```python
from build123d import *

# Parameters (mm, degrees)
SKETCH_1_R          = 2.55
EXTRUDE_1_DEPTH     = 10
SKETCH_2_W          = 40
SKETCH_2_H          = 20
EXTRUDE_2_DEPTH     = 3
EXTRUDE_3_DEPTH     = 3
CUT_EXTRUDE_1_DEPTH = 10
SKETCH_5_R          = 3
CUT_EXTRUDE_2_DEPTH = 10
SKETCH_6_R          = 3
SKETCH_6_R_2        = 4.25
EXTRUDE_4_DEPTH     = 3
FILLET_1_R          = 1.5
SKETCH_7_R          = 6
SKETCH_7_R_2        = 3
EXTRUDE_5_DEPTH     = 5
SKETCH_8_R          = 8.25
EXTRUDE_6_DEPTH     = 5
FILLET_3_R          = 1.5


with BuildPart() as part:
    # 草图1 → 凸台-拉伸1 (new body)
    with BuildSketch(Plane.XY):
        Polygon((-20, 0), (-20, -6.9), (-18.2, -6.9), (-18.2, -4.5), (-16.560660172, -4.5), (-13.9, -7.160660172), (-13.9, -12.839339828), (-16.560660172, -15.5), (-18.2, -15.5), (-18.2, -13.1), (-20, -13.1), (-20, -20), (-13.1, -20), (-13.1, -18.2), (-15.5, -18.2), (-15.5, -16.560660172), (-12.839339828, -13.9), (-7.160660172, -13.9), (-4.5, -16.560660172), (-4.5, -18.2), (-6.9, -18.2), (-6.9, -20), (0, -20), (6.9, -20), (6.9, -18.2), (4.5, -18.2), (4.5, -16.560660172), (7.160660172, -13.9), (12.839339828, -13.9), (15.5, -16.560660172), (15.5, -18.2), (13.1, -18.2), (13.1, -20), (20, -20), (20, -13.1), (18.2, -13.1), (18.2, -15.5), (16.560660172, -15.5), (13.9, -12.839339828), (13.9, -7.160660172), (16.560660172, -4.5), (18.2, -4.5), (18.2, -6.9), (20, -6.9), (20, 0), (13.1, 0), (13.1, -1.8), (15.5, -1.8), (15.5, -3.439339828), (12.839339828, -6.1), (7.160660172, -6.1), (4.5, -3.439339828), (4.5, -1.8), (6.9, -1.8), (6.9, 0), (0, 0), (-6.9, 0), (-6.9, -1.8), (-4.5, -1.8), (-4.5, -3.439339828), (-7.160660172, -6.1), (-12.839339828, -6.1), (-15.5, -3.439339828), (-15.5, -1.8), (-13.1, -1.8), (-13.1, 0), align=None)
        with Locations((-10, -10)):
            Circle(SKETCH_1_R, mode=Mode.SUBTRACT)
        with Locations((10, -10)):
            Circle(SKETCH_1_R, mode=Mode.SUBTRACT)
        Polygon((-3.439339828, -4.5), (-6.1, -7.160660172), (-6.1, -12.839339828), (-3.439339828, -15.5), (-3.439339828, -18.2), (3.439339828, -18.2), (3.439339828, -15.5), (6.1, -12.839339828), (6.1, -7.160660172), (3.439339828, -4.5), (3.439339828, -1.8), (-3.439339828, -1.8), align=None, mode=Mode.SUBTRACT)
    extrude(amount=EXTRUDE_1_DEPTH)

    # 草图2 → 凸台-拉伸2 (add)
    with BuildSketch(Plane.XY.offset(10)):
        with Locations((0, -10)):
            Rectangle(SKETCH_2_W, SKETCH_2_H)
    extrude(amount=EXTRUDE_2_DEPTH)

    # 草图3 → 凸台-拉伸3 (add)
    with BuildSketch(Plane(origin=(0, 0, 10), x_dir=(-1, 0, 0), z_dir=(0, 0, -1))):
        Polygon((-13.1, -20), (-6.9, -20), (-6.9, -18.2), (-4.5, -18.2), (-4.5, -16.560660172), (-7.160660172, -13.9), (-12.839339828, -13.9), (-15.5, -16.560660172), (-15.5, -18.2), (-13.1, -18.2), align=None)
        Polygon((-20, -6.9), (-20, -13.1), (-18.2, -13.1), (-18.2, -15.5), (-16.560660172, -15.5), (-13.9, -12.839339828), (-13.9, -7.160660172), (-16.560660172, -4.5), (-18.2, -4.5), (-18.2, -6.9), align=None)
        Polygon((-6.9, 0), (-13.1, 0), (-13.1, -1.8), (-15.5, -1.8), (-15.5, -3.439339828), (-12.839339828, -6.1), (-7.160660172, -6.1), (-4.5, -3.439339828), (-4.5, -1.8), (-6.9, -1.8), align=None)
        Polygon((6.9, -20), (13.1, -20), (13.1, -18.2), (15.5, -18.2), (15.5, -16.560660172), (12.839339828, -13.9), (7.160660172, -13.9), (4.5, -16.560660172), (4.5, -18.2), (6.9, -18.2), align=None)
        Polygon((20, -13.1), (20, -6.9), (18.2, -6.9), (18.2, -4.5), (16.560660172, -4.5), (13.9, -7.160660172), (13.9, -12.839339828), (16.560660172, -15.5), (18.2, -15.5), (18.2, -13.1), align=None)
        Polygon((13.1, 0), (6.9, 0), (6.9, -1.8), (4.5, -1.8), (4.5, -3.439339828), (7.160660172, -6.1), (12.839339828, -6.1), (15.5, -3.439339828), (15.5, -1.8), (13.1, -1.8), align=None)
    extrude(amount=EXTRUDE_3_DEPTH)

    # 草图4 → 切除-拉伸1 (cut)
    with BuildSketch(Plane(origin=(0, 0, 0), x_dir=(-1, 0, 0), z_dir=(0, 0, -1))):
        Polygon((6.9, 0), (-6.9, 0), (-6.9, -1.8), (-4.5, -1.8), (-4.5, -3.439339828), (-7.160660172, -6.1), (-12.839339828, -6.1), (-15.5, -3.439339828), (-15.5, -1.8), (-13.1, -1.8), (-13.1, 0), (-20, 0), (-20, -6.9), (-18.2, -6.9), (-18.2, -4.5), (-16.560660172, -4.5), (-13.9, -7.160660172), (-13.9, -12.839339828), (-16.560660172, -15.5), (-18.2, -15.5), (-18.2, -13.1), (-20, -13.1), (-20, -20), (-13.1, -20), (-13.1, -18.2), (-15.5, -18.2), (-15.5, -16.560660172), (-12.839339828, -13.9), (-7.160660172, -13.9), (-4.5, -16.560660172), (-4.5, -18.2), (-6.9, -18.2), (-6.9, -20), (6.9, -20), (6.9, -18.2), (4.5, -18.2), (4.5, -16.560660172), (7.160660172, -13.9), (12.839339828, -13.9), (15.5, -16.560660172), (15.5, -18.2), (13.1, -18.2), (13.1, -20), (20, -20), (20, -13.1), (18.2, -13.1), (18.2, -15.5), (16.560660172, -15.5), (13.9, -12.839339828), (13.9, -7.160660172), (16.560660172, -4.5), (18.2, -4.5), (18.2, -6.9), (20, -6.9), (20, 0), (13.1, 0), (13.1, -1.8), (15.5, -1.8), (15.5, -3.439339828), (12.839339828, -6.1), (7.160660172, -6.1), (4.5, -3.439339828), (4.5, -1.8), (6.9, -1.8), align=None)
    extrude(amount=-CUT_EXTRUDE_1_DEPTH, mode=Mode.SUBTRACT)

    # 草图5 → 切除-拉伸2 (cut)
    with BuildSketch(Plane(origin=(0, 0, 10), x_dir=(-1, 0, 0), z_dir=(0, 0, -1))):
        with Locations((-10, -10)):
            Circle(SKETCH_5_R)
        with Locations((10, -10)):
            Circle(SKETCH_5_R)
    extrude(amount=-CUT_EXTRUDE_2_DEPTH, mode=Mode.SUBTRACT)

    # 草图6 → 凸台-拉伸4 (add)
    with BuildSketch(Plane.XY.offset(13)):
        Polygon((-20, 0), (20, 0), (20, 35), (0, 35), (-20, 35), align=None)
        with Locations((-10, 10.36)):
            Circle(SKETCH_6_R, mode=Mode.SUBTRACT)
        with Locations((10, 10.36)):
            Circle(SKETCH_6_R, mode=Mode.SUBTRACT)
        with Locations((0, 25)):
            Circle(SKETCH_6_R_2, mode=Mode.SUBTRACT)
    extrude(amount=-EXTRUDE_4_DEPTH)

    # 圆角1
    fillet_1_edges = [part.edges().sort_by_distance(p)[0] for p in [
        (20, -20, 11.5),
        (-20, -20, 11.5),
        (-20, 35, 11.5),
        (20, 35, 11.5),
    ]]
    fillet(fillet_1_edges, radius=FILLET_1_R)

    # 草图7 → 凸台-拉伸5 (add)
    # profile 1 of 2: a face of its own
    with BuildSketch(Plane(origin=(0, 0, 10), x_dir=(-1, 0, 0), z_dir=(0, 0, -1))):
        with Locations(Location((-10, 10.36, 0), (0, 0, 180))):
            Circle(SKETCH_7_R)
        with Locations(Location((-10, 10.36, 0), (0, 0, 180))):
            Circle(SKETCH_7_R_2, mode=Mode.SUBTRACT)
    # profile 2 of 2: a face of its own
    with BuildSketch(Plane(origin=(0, 0, 10), x_dir=(-1, 0, 0), z_dir=(0, 0, -1))):
        with Locations(Location((10, 10.36, 0), (0, 0, 180))):
            Circle(SKETCH_7_R)
        with Locations(Location((10, 10.36, 0), (0, 0, 180))):
            Circle(SKETCH_7_R_2, mode=Mode.SUBTRACT)
    extrude(amount=EXTRUDE_5_DEPTH)

    # 草图8 → 凸台-拉伸6 (add)
    with BuildSketch(Plane(origin=(0, 0, 10), x_dir=(-1, 0, 0), z_dir=(0, 0, -1))):
        with BuildLine():
            Line((-4.582575695, 35), (4.582575695, 35))
            ThreePointArc((4.582575695, 35), (0, 14), (-4.582575695, 35))
        make_face()
        with Locations((0, 25)):
            Circle(SKETCH_8_R, mode=Mode.SUBTRACT)
    extrude(amount=EXTRUDE_6_DEPTH)

    # 圆角3
    # the kernel refuses this fillet: 1.5 mm, written as the material it adds along each edge
    with BuildSketch(Plane(origin=(10, 10.36, 10), x_dir=(1, 0, 0), z_dir=(0, 1, 0))) as fillet_3_piece_1:
        with BuildLine():
            CenterArc((6 + FILLET_3_R, FILLET_3_R), FILLET_3_R, 180, 90)
            Line((6, FILLET_3_R), (6 - FILLET_3_R * 0.02, FILLET_3_R))
            Line((6 - FILLET_3_R * 0.02, FILLET_3_R), (6 - FILLET_3_R * 0.02, -FILLET_3_R * 0.02))
            Line((6 - FILLET_3_R * 0.02, -FILLET_3_R * 0.02), (6 + FILLET_3_R, -FILLET_3_R * 0.02))
            Line((6 + FILLET_3_R, -FILLET_3_R * 0.02), (6 + FILLET_3_R, 0))
        make_face()
    revolve(axis=Axis((10, 10.36, 10), (0, 0, -1)))
    with BuildSketch(Plane(origin=(-10, 10.36, 10), x_dir=(1, 0, 0), z_dir=(0, 1, 0))) as fillet_3_piece_2:
        with BuildLine():
            CenterArc((6 + FILLET_3_R, FILLET_3_R), FILLET_3_R, 180, 90)
            Line((6, FILLET_3_R), (6 - FILLET_3_R * 0.02, FILLET_3_R))
            Line((6 - FILLET_3_R * 0.02, FILLET_3_R), (6 - FILLET_3_R * 0.02, -FILLET_3_R * 0.02))
            Line((6 - FILLET_3_R * 0.02, -FILLET_3_R * 0.02), (6 + FILLET_3_R, -FILLET_3_R * 0.02))
            Line((6 + FILLET_3_R, -FILLET_3_R * 0.02), (6 + FILLET_3_R, 0))
        make_face()
    revolve(axis=Axis((-10, 10.36, 10), (0, 0, -1)))
    with BuildSketch(Plane(origin=(0, 25, 10), x_dir=(-0.08704252820230896, 0.9962045965985854, 0), z_dir=(0.9962045965985854, 0.08704252820230896, 0))) as fillet_3_piece_3_section:
        with BuildLine():
            CenterArc((11 + FILLET_3_R, -FILLET_3_R), FILLET_3_R, 90, 90)
            Line((11, -FILLET_3_R), (11 - FILLET_3_R * 0.02, -FILLET_3_R))
            Line((11 - FILLET_3_R * 0.02, -FILLET_3_R), (11 - FILLET_3_R * 0.02, FILLET_3_R * 0.02))
            Line((11 - FILLET_3_R * 0.02, FILLET_3_R * 0.02), (11 + FILLET_3_R, FILLET_3_R * 0.02))
            Line((11 + FILLET_3_R, FILLET_3_R * 0.02), (11 + FILLET_3_R, 0))
        make_face()
    fillet_3_piece_3 = revolve(axis=Axis((0, 25, 10), (0, 0, 1)), revolution_arc=350.013022923, mode=Mode.PRIVATE)
    fillet_3_piece_3 = split(fillet_3_piece_3, bisect_by=Plane(origin=(0, 35, 9.583684296), z_dir=(0, -1, 0)), keep=Keep.TOP, mode=Mode.PRIVATE)
    add(fillet_3_piece_3)


solid = part.part
```
Input: part model. Units: mm. Frame: model coordinates. A direction names the side the tool comes from. Coordinates: 2 decimals unless noted, no trailing zeros. Loops run counter-clockwise (first coordinate to the right, second up) from the corner with the lowest first, then second, coordinate; pieces in that order, holes last. Notation, with made-up numbers: M 43,4.5 L 90,4.5 A15 cw 90,8.5 Z; hole C -39.75,57.5 d8. An arc over 180 degrees is marked long. One line per item, written item: value.
(1) Reachability of faces 1 (the flat face through (18.2, -6, 8)), 2 (the flat face through (-6.9, -1, 8)), 3 (the flat face through (10, -3, 7)) from +Z, -Z, +X, -X, +Y, -Y: full face, straight path, thin tool, end or side. Return the list, or none.
Filled in:
face 1: -Z, +X, +Y
face 2: -Z
face 3: -Z, +X, -X, -Y
(2) Section A-A (y = -10). Output: boundary loops of the cut face in (x, z).
Filled in:
outline: M -20,7 L -13.9,7 L -13.9,10 L -13,10 L -13,13 L -20,13 Z; M -7,10 L 7,10 L 7,13 L -7,13 Z; M 13,10 L 13.9,10 L 13.9,7 L 20,7 L 20,13 L 13,13 Z
(3) Section D-D (z = 12). Output: boundary loops of the cut face in (x, y), and give its area (3 significant figures).
Filled in:
outline: M -20,-18.5 A1.5 ccw -18.5,-20 L 18.5,-20 A1.5 ccw 20,-18.5 L 20,33.5 A1.5 ccw 18.5,35 L -18.5,35 A1.5 ccw -20,33.5 Z; hole C -10,-10 d6; hole C -10,10.36 d6; hole C 0,25 d8.5; hole C 10,-10 d6; hole C 10,10.36 d6
area: 2,030 mm^2
(4) Pin query (flat end, axial travel): pin 1 (12 mm diameter, centred on x = 0.5, y = 24.5, fed in from -Z); pin 2 (6.5 mm diameter, centred on x = 17, y = -12.5, fed in from -Z); pin 3 (1.3 mm diameter, centred on x = 17.5, z = 9, fed in from -Y). Return the tip coordinate at first contact, or that it passes through.
Filled in:
pin 1: z = 10
pin 2: z = 7
pin 3: y = -15.5
(5) Section C-C (y = 25). Output: boundary loops of the cut face in (x, z).
Filled in:
outline: M -20,10 L -12.5,10 A1.5 cw -11,8.5 L -11,5 L -8.25,5 L -8.25,10 L -4.25,10 L -4.25,13 L -20,13 Z; M 4.25,10 L 8.25,10 L 8.25,5 L 11,5 L 11,8.5 A1.5 cw 12.5,10 L 20,10 L 20,13 L 4.25,13 Z
(6) Line query: line 1 along Y through (x, z) = (-10, 12.2); line 2 along X through (y, z) = (10.36, 8.6); line 3 along Y through (x, z) = (0, 6.1). Output: solid intervals per line, ascending. Write a range as from..to.
Filled in:
line 1: -20..-13, -7..7.36, 13.36..35
line 2: -16..-13, -7..-4, 4..7, 13..16
line 3: 14..16.75, 33.25..35
(7) Section B-B (x = 0). Output: boundary loops of the cut face in (y, z), and give its area (3 significant figures).
Filled in:
outline: M -20,10 L 12.5,10 A1.5 cw 14,8.5 L 14,5 L 16.75,5 L 16.75,10 L 20.75,10 L 20.75,13 L -20,13 Z; M 29.25,10 L 33.25,10 L 33.25,5 L 35,5 L 35,13 L 29.25,13 Z
area: 162 mm^2
(8) Pull-direction query (Y, two-part tool) for faces 4 (the flat face through (-19, -13.1, 8)), 5 (the flat face through (14, -1.8, 8)), 6 (the flat face through (4.5, -17, 8)); classes: +Y half, -Y half, draft (parallel to the pull), parting line (faces both ways), or undercut.
Filled in:
face 4: -Y half
face 5: undercut
face 6: draft
